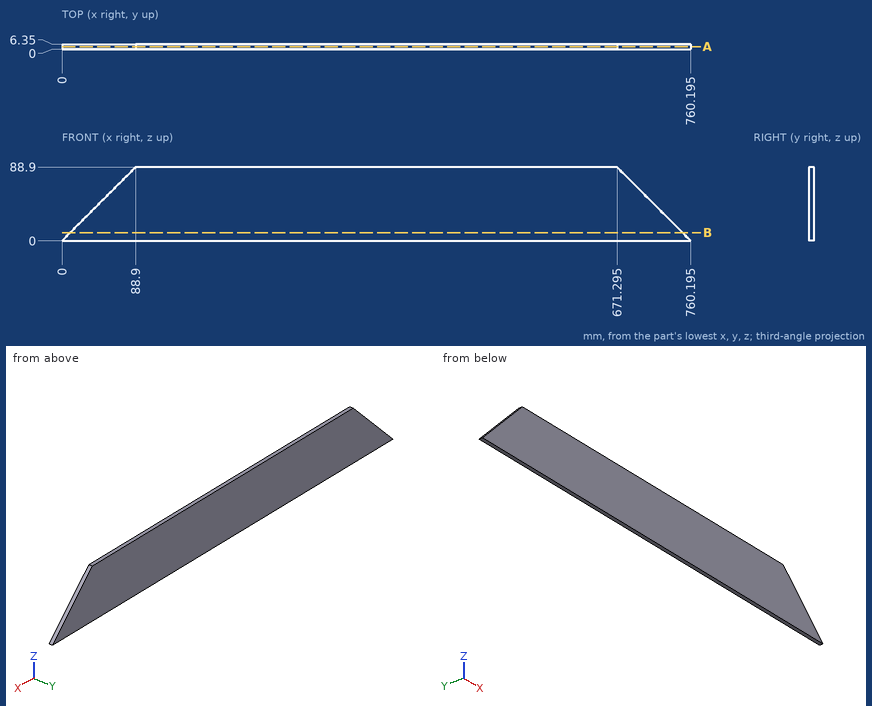
Drawing for the job (mm, zero at the part's lowest x, y, z). Give positions to 0.01 mm unless a question says otherwise; leave off trailing zeros. Write each loop counter-clockwise with the first axis right and the second up, starting at its lowest first coordinate (ties: lowest second). Pieces come first, ordered by that corner, then holes. Notation, with made-up numbers: (-5, 36.25) - (16, 36.25) arc R27 ccw to (16, 56.25) - close; hole circle Ø6 at (-20, 55.25). An arc over 180 degrees is marked (long way). Answer as CSV lines item,"result".
Q1. Band-saw the part on B-B (z = 10). Give the cut face in (x, y) (3 decimals).
Result set:
outline,"(10, 0) - (750.195, 0) - (750.195, 6.35) - (10, 6.35) - close"
Q2. Band-saw the part on A-A (y = 3.25). Give the cut face in (x, z) (3 decimals).
Result set:
outline,"(0, 0) - (760.195, 0) - (671.295, 88.9) - (88.9, 88.9) - close"
Q3. Drill centre lines: line 1 (X direction, y = 1, z = 65) (1 decimal); line 2 (X direction, y = 2.75, z = 51) (1 decimal); line 3 (Z direction, x = 714, y = 2.75) (1 decimal). Where is each one in solid material? Low to high. Write a range as from..to.
Result set:
line 1,"65..695.2"
line 2,"51..709.2"
line 3,"0..46.2"
Q4. Flat gauge pins, fed straight in: pin 1 Ø3 at (y, z) = (5, 61) entering from -X; pin 2 Ø2 at (y, z) = (1.5, 11.5) entering from +X (1 decimal). Where does each tip first touch, or does it go through?
Result set:
pin 1,"x = 59.5"
pin 2,"x = 749.7"
